Verification items for the finished model (mm, model axes). A direction names the side the tool comes from. Coordinates: 2 decimals unless noted, no trailing zeros. Order: outer loops, then holes, each group sorted by start corner. A loop starts at its lowest first (then second) coordinate and runs counter-clockwise, first axis right, second up. Notation, with made-up numbers: (-9.5, 12.25) - (45.5, 12.25) arc R24 ccw to (45.5, 23.25) - close; hole circle Ø3 at (78.25, 80.5). An arc over 180 degrees is marked (long way). Answer as CSV lines item,"result". Start each with the question number.
1. Section check B-B (y = -45.5). Record the cut outline in (x, z).
2. Mould release check, pull along X, two halves, no side actions. Record for faces 3 (the flat face through (0, -40, 168.832)), 4 (the flat face through (30, -40, 42)), 5 (the flat face through (0, -39, 167.832)), 6 (the flat face through (-30, -40, 42)): pulls with the +X half, pulls with the -X half, needs draft (parallel to the pull), parting line crosses it, or undercut.
3. Go/stop test with flat-tipped pins: pin 1 (4 mm diameter, centred on x = 5.5, z = 14, fed in from -Y); pin 2 (3 mm diameter, centred on x = -15.5, y = -26.5, fed in from -Z). Record where each tip stops, or that it passes through.
4. Set-up check for faces 1 (the flat face through (0, 1.5, 46)), 2 (the flat face through (29, -39, 46)): record each of +Z, -Z, +X, -X, +Y, -Y from which the full face is reachable in a straight line by a thin tool's end or side.
5. Material ranges on L1, parallel to X at y = -73, z = 77.5; L2, parallel to Z at x = 26, y = -20.5; L3, parallel to Y at x = -17.5, z = -12.5, recorded low to high. Write a range as [from, to].
6. Section check A-A (z = 124.5). Record the cut outline in (x, y).
7. Section check C-C (x = 13). Record the cut outline in (y, z), and give its area (3 significant figures).
from build123d import *

# Parameters (mm, degrees)
F1_DEPTH = 80
F2_W     = 60
F2_H     = 250
F3_DEPTH = 1.5


# Not quite as in the source:
# - a feature of the source that left no trace in its solid (it failed there, or was rolled back) is left out


with BuildPart() as f1:
    # F0 (on Front) → F1 (new body)
    with BuildSketch(Plane.XZ):
        Polygon((30, 168.8320699929), (-30, 168.8320699929), (-30, -81.1679300071), (-25, -81.1679300071), (-25, -79.1679300071), (-29, -79.1679300071), (-29, 167.8320699929), (29, 167.8320699929), (29, -79.1679300071), (25, -79.1679300071), (25, -81.1679300071), (30, -81.1679300071), align=None)
    extrude(amount=F1_DEPTH)

    # F2 (on face) → F3 (join)
    with BuildSketch(Plane(origin=(0, 0, 0), x_dir=(-1, 0, 0), z_dir=(0, 1, 0))):
        with Locations((0, 43.8320699929)):
            Rectangle(F2_W, F2_H)
    extrude(amount=F3_DEPTH)


solid = f1.part
Evaluation:
1,outline,"(-30, -81.17) - (-25, -81.17) - (-25, -79.17) - (-29, -79.17) - (-29, 167.83) - (29, 167.83) - (29, -79.17) - (25, -79.17) - (25, -81.17) - (30, -81.17) - (30, 168.83) - (-30, 168.83) - close"
2,face 3,"needs draft"
2,face 4,"pulls with the +X half"
2,face 5,"undercut"
2,face 6,"pulls with the -X half"
3,pin 1,"stops at y = 0"
3,pin 2,"stops at z = 167.83"
4,face 1,"+Z, -Z, +X, -X, +Y"
4,face 2,"-Y"
5,L1,"x = [-30, -29], [29, 30]"
5,L2,"z = [-81.17, -79.17], [167.83, 168.83]"
5,L3,"y = [0, 1.5]"
6,outline,"(-30, -80) - (-29, -80) - (-29, 0) - (29, 0) - (29, -80) - (30, -80) - (30, 1.5) - (-30, 1.5) - close"
7,outline,"(-80, 167.83) - (0, 167.83) - (0, -81.17) - (1.5, -81.17) - (1.5, 168.83) - (-80, 168.83) - close"
7,area,"455 mm²"
